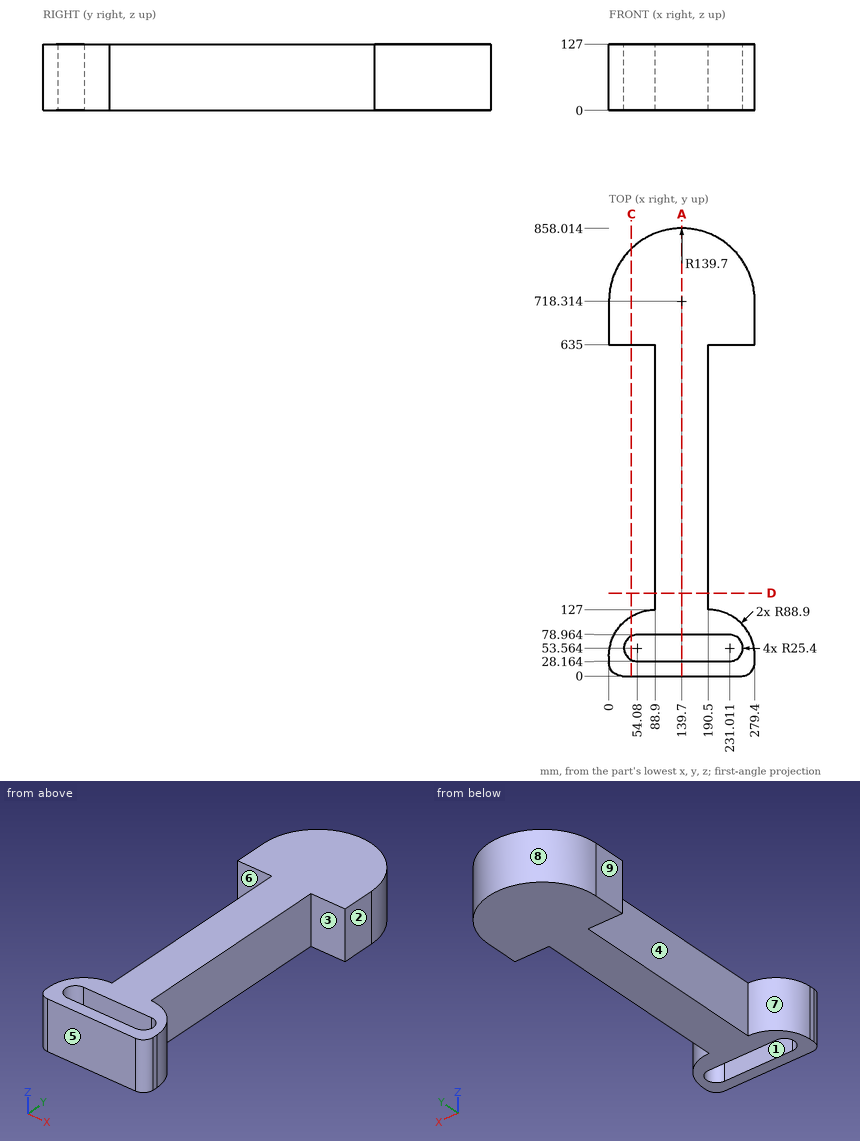
Check sheet for the drawn part. Datum: minimum x, y, z corner. Units: mm. A direction names the side the tool comes from. Coordinates: 2 decimals unless noted, no trailing zeros. Loops run counter-clockwise (first coordinate to the right, second up) from the corner with the lowest first, then second, coordinate; pieces in that order, holes last. Notation, with made-up numbers: (86.25, 45.5) -> (108.25, 45.5) arc R23 ccw to (108.25, 61.5) -> close; hole circle Ø3 at (0, 50). An arc over 180 degrees is marked (long way). Answer as CSV lines item,"result".
1) Thickness scan on L1, parallel to Y at x = 221, z = 108.5 (1 decimal); L2, parallel to Y at x = 207, z = 99 (1 decimal); L3, parallel to Y at x = 136.5, z = 68 (1 decimal). Record the ranges inside material, lowest first. Write a range as from..to.
Found:
L1,"y = 0..28.2, 79..121.6, 635..831.9"
L2,"y = 0..28.2, 79..125.5, 635..840.7"
L3,"y = 0..28.2, 79..858"
2) Cross-section at A-A, the plane x = 139.7. Record the cut outline in (y, z) (1 decimal).
Found:
outline,"(0, 0) -> (28.2, 0) -> (28.2, 127) -> (0, 127) -> close; (79, 0) -> (858, 0) -> (858, 127) -> (79, 127) -> close"
3) Release check for a two-part mould opening along Y. For the marked faces 6, 7, 8 and 9 record: +Y half, -Y half, draft (parallel to the pull), parting line (faces both ways), or undercut.
Found:
face 6,"undercut"
face 7,"undercut"
face 8,"+Y half"
face 9,"draft"
4) Tool access check on the marked faces 1, 2, 3, 4 and 5. Record the directions out of +Z, -Z, +X, -X, +Y, -Y that give a thin tool (end or side, any length) a straight path to the whole face; none if there is none.
Found:
face 1,"+Z, -Z"
face 2,"+Z, -Z, +X, +Y, -Y"
face 3,"+Z, -Z, +X"
face 4,"+Z, -Z, -X"
face 5,"+Z, -Z, +X, -X, -Y"
5) Cross-section at D-D, the plane y = 159. Record the cut outline in (x, z).
Found:
outline,"(88.9, 0) -> (190.5, 0) -> (190.5, 127) -> (88.9, 127) -> close"
6) Cross-section at C-C, the plane x = 43. Record the cut outline in (y, z) (1 decimal), then the cut area to 3 significant figures.
Found:
outline,"(0, 0) -> (30.7, 0) -> (30.7, 127) -> (0, 127) -> close; (76.4, 0) -> (114.2, 0) -> (114.2, 127) -> (76.4, 127) -> close; (635, 0) -> (819.1, 0) -> (819.1, 127) -> (635, 127) -> close"
area,"32,100 mm2"
7) Depth check by flat-ended pin: pin 1 (5 mm diameter, centred on x = 236, z = 100.5, fed in from -Y); pin 2 (12 mm diameter, centred on y = 336, z = 43, fed in from +X); pin 3 (10 mm diameter, centred on y = 93, z = 24.5, fed in from -X) (1 decimal); pin 4 (10 mm diameter, centred on x = 197, z = 97.5, fed in from +Y) (1 decimal). Enter the tip coordinate at first touch or a pass-through.
Found:
pin 1,"stops at y = 0"
pin 2,"stops at x = 190.5"
pin 3,"stops at x = 15.3"
pin 4,"stops at y = 847.9"
